Geometry: final body of the model. Coordinates: model frame, mm. Coordinates: 2 decimals unless noted, no trailing zeros. Loops run counter-clockwise (first coordinate to the right, second up) from the corner with the lowest first, then second, coordinate; pieces in that order, holes last. Notation, with made-up numbers: (87, -12.75) -> (109, -12.75) arc R21 cw to (109, 9.25) -> close; hole circle Ø2 at (64, -11). An arc over 180 degrees is marked (long way). One line per item, written item: value. Start each with the question number.
from build123d import *

# Parameters (mm, degrees)
F1_DEPTH = 3.175
F2_SIZE  = 3.17499


# Not quite as in the source:
# - a fillet or chamfer is up to 0.001 mm smaller than in the source, because OpenCascade refuses the exact size


with BuildPart() as f1:
    # F0 (on Top) → F1 (new body, symmetric)
    with BuildSketch(Plane.XY):
        with BuildLine():
            ThreePointArc((22.3162673387, -60.1211733557), (19.6694953196, 9.2531133838), (0, 75.8332006216))
            ThreePointArc((0, 75.8332006216), (-19.8842446441, 9.2801862209), (-22.7369976658, -60.1211733557))
            Line((-22.7369976658, -60.1211733557), (22.3162673387, -60.1211733557))
        make_face()
    extrude(amount=F1_DEPTH, both=True)

    # F2 (size 3.175 in the source; OpenCascade refuses exactly that, so slightly less here)
    f2_edges = [f1.edges().sort_by_distance(p)[0] for p in [
        (-0.210365, -60.121173, 3.175),
        (19.669495, 9.253113, 3.175),
        (-19.884245, 9.280186, 3.175),
        (-0.210365, -60.121173, -3.175),
        (19.669495, 9.253113, -3.175),
        (-19.884245, 9.280186, -3.175),
    ]]
    chamfer(f2_edges, length=F2_SIZE)


solid = f1.part
1. Section A-A on z = -1.25. Return the cut outline in (x, y).
2. Pin query (flat end, axial travel): pin 1 Ø2 at (y, z) = (27.5, 0.5) entering from +X. Return the tip coordinate at first contact, or that it passes through.
3. Line query: L1, parallel to X at y = 9, z = -0.5; L2, parallel to Z at x = -18, y = 1.5; L3, parallel to X at y = 29.5, z = -1.5. Output: solid intervals per line, ascending. Write a range as [from, to].
Checks:
1. outline: (-21.58, -58.87) -> (21.17, -58.87) arc R278.15 ccw to (0, 72.68) arc R278.15 ccw to start
2. pin 1: x = 16.25
3. L1: [-19.42, 19.2]
3. L2: [-3.04, 3.04]
3. L3: [-14.19, 14.03]
